The model under review builds one solid part; all positions refer to its coordinate system, in mm. A direction names the side the tool comes from. Give positions to 0.01 mm unless a question says otherwise; leave off trailing zeros. Write each loop counter-clockwise with the first axis right and the second up, starting at its lowest first coordinate (ties: lowest second). Pieces come first, ordered by that corner, then holes. Notation, with made-up numbers: M 19,24 L 33,24 A19 ccw 33,32 Z; hole C 77.25,-27 d4. An arc over 180 degrees is marked long. Write item = value, one per line. Start each with the question number.
```python
from build123d import *

# Parameters (mm, degrees)
SKETCH1_W                 = 260
SKETCH1_H                 = 80
BOSS_EXTRUDE1_DEPTH       = 100
SKETCH2_W                 = 250
SKETCH2_H                 = 70.000000188
INSIDE_DEPTH              = 90
SKETCH8_W                 = 9
SKETCH8_H                 = 9
WIRE_HOLES_DEPTH          = 23
SKETCH12_W                = 66
SKETCH12_H                = 4
VENTALATION_DEPTH         = 15
SKETCH14_W                = 66
SKETCH14_H                = 4
VENTALATION_2_DEPTH       = 10
SKETCH16_W                = 66
SKETCH16_H                = 4
VENTALATION_3_DEPTH       = 10
SKETCH20_W                = 34
SKETCH20_H                = 30
COMMAND_STRIP_FRONT_DEPTH = 1
SKETCH21_W                = 30
SKETCH21_H                = 34.000000188
COMMAND_STRIP_RIGHT_DEPTH = 1
SKETCH22_W                = 30
SKETCH22_H                = 34.000000188
BOSS_EXTRUDE4_DEPTH       = 1


with BuildPart() as part:
    # Sketch1 → Boss-Extrude1 (new body)
    with BuildSketch(Plane(origin=(0, 0, 0), x_dir=(1, 0, 0), z_dir=(0, 1, 0))):
        Rectangle(SKETCH1_W, SKETCH1_H)
    extrude(amount=BOSS_EXTRUDE1_DEPTH)

    # Sketch2 → inside (cut)
    with BuildSketch(Plane.XZ):
        Rectangle(SKETCH2_W, SKETCH2_H)
    extrude(amount=-INSIDE_DEPTH, mode=Mode.SUBTRACT)

    # Sketch8 → Wire holes (cut)
    with BuildSketch(Plane.XY.offset(40)):
        with Locations((-71, 44.5)):
            Rectangle(SKETCH8_W, SKETCH8_H)
        with Locations((-42, 44.5)):
            Rectangle(SKETCH8_W, SKETCH8_H)
        with Locations((46.75, 44.5)):
            Rectangle(SKETCH8_W, SKETCH8_H)
    extrude(amount=-WIRE_HOLES_DEPTH, mode=Mode.SUBTRACT)

    # Sketch12 → Ventalation (cut)
    with BuildSketch(Plane(origin=(130, 0, 0), x_dir=(0, 0, -1), z_dir=(1, 0, 0))):
        with Locations((0, 84)):
            Rectangle(SKETCH12_W, SKETCH12_H)
    extrude(amount=-VENTALATION_DEPTH, mode=Mode.SUBTRACT)

    # Sketch14 → Ventalation 2 (cut)
    with BuildSketch(Plane(origin=(130, 0, 0), x_dir=(0, 0, -1), z_dir=(1, 0, 0))):
        with Locations((0, 75)):
            Rectangle(SKETCH14_W, SKETCH14_H)
    extrude(amount=-VENTALATION_2_DEPTH, mode=Mode.SUBTRACT)

    # Sketch16 → Ventalation 3 (cut)
    with BuildSketch(Plane(origin=(130, 0, 0), x_dir=(0, 0, -1), z_dir=(1, 0, 0))):
        with Locations((0, 66)):
            Rectangle(SKETCH16_W, SKETCH16_H)
    extrude(amount=-VENTALATION_3_DEPTH, mode=Mode.SUBTRACT)

    # Sketch20 → Command Strip front (add)
    with BuildSketch(Plane.XZ):
        with Locations((0, -50.000000094)):
            Rectangle(SKETCH20_W, SKETCH20_H)
    extrude(amount=COMMAND_STRIP_FRONT_DEPTH)

    # Sketch21 → Command strip right (add)
    with BuildSketch(Plane.XZ):
        with Locations((-140, 0)):
            Rectangle(SKETCH21_W, SKETCH21_H)
    extrude(amount=COMMAND_STRIP_RIGHT_DEPTH)

    # Sketch22 → Boss-Extrude4 (add)
    with BuildSketch(Plane.XZ):
        with Locations((140, 0)):
            Rectangle(SKETCH22_W, SKETCH22_H)
    extrude(amount=BOSS_EXTRUDE4_DEPTH)


solid = part.part
```
Item 1: We need section A-A, the plane y = 27. Write out the cut boundary in (x, z).
Item 2: The part is to be moulded in two halves that separate along Z. For faces 5 (the flat face through (77, 0, -36)), 6 (the flat face through (-2, 49, -40)), 7 (the flat face through (-2, 90, 0)), 8 (the flat face through (125, 25, 0)), say which applies: released by +Z, released by -Z, zero draft, split by the parting line, or undercut.
Item 3: We need section B-B, the plane z = 29. Write out the cut boundary in (x, y).
Item 4: Clearance check with flat-ended pins moving along their axes: P1, Ø7, axis at x = 101, z = -29.5, coming from the -Y side; P2, Ø1.1, axis at x = 133.5, y = -0.5, coming from the +Z side; P3, Ø2.5, axis at y = 44.5, z = 38, coming from the -X side. State where each tip first meets the part, or that it passes through.
Item 5: We need section D-D, the plane z = -57. Write out the cut boundary in (x, y), and give its area (3 significant figures).
Item 6: To check wall thickness, follow probe 1 along Z at (x, y) = (-72, 78.5); probe 2 along X at (y, z) = (21, -29); probe 3 along X at (y, z) = (92.5, 10.5). State the ranges of each line that lie inside material, in increasing order. Write a range as [from, to].
Item 7: For faces 1 (the flat face through (-2, 44, 35)), 2 (the flat face through (-19.9, 0, 35.3)), 3 (the flat face through (-143, 0, 0)), 4 (the flat face through (0, 0, -52)), list the 3-axis set-ups (+Z, -Z, +X, -X, +Y, -Y) from which the entire face can be reached by the end or side of a thin tool; tool diameter is ignored.
Item 8: We need section C-C, the plane x = -62. Write out the cut boundary in (y, z).
Worked out:
q1.outline = M -130,-40 L 130,-40 L 130,40 L -130,40 Z; hole M -125,-35 L 125,-35 L 125,35 L -125,35 Z
q2.face_5 = zero draft
q2.face_6 = released by -Z
q2.face_7 = undercut
q2.face_8 = undercut
q3.outline = M -130,0 L -125,0 L -125,90 L 125,90 L 125,86 L 130,86 L 130,100 L -130,100 Z; M 125,0 L 130,0 L 130,64 L 125,64 Z; M 125,68 L 130,68 L 130,73 L 125,73 Z; M 125,77 L 130,77 L 130,82 L 125,82 Z
q4.P1 = 90
q4.P2 = 17
q4.P3 = -130
q5.outline = M -17,-1 L 17,-1 L 17,0 L -17,0 Z
q5.area = 34.0 mm²
q6.probe_1 = [-40, -35], [35, 40]
q6.probe_2 = [-130, -125], [125, 130]
q6.probe_3 = [-130, 130]
q7.face_1 = -Y
q7.face_2 = +Z, +X, -X, -Y
q7.face_3 = +Z, -Z, -X, +Y
q7.face_4 = -Z, +X, -X, +Y
q8.outline = M 0,-40 L 100,-40 L 100,40 L 0,40 L 0,35 L 90,35 L 90,-35 L 0,-35 Z
